from build123d import *

# Parameters (mm, degrees)
F1_DEPTH = 2.4
F2_DEPTH = 8
F3_W     = 64.007707
F3_H     = 6.8
F4_DEPTH = 25
F5_W     = 73.7
F5_H     = 31.871149
F6_DEPTH = 25


with BuildPart() as f1:
    # F0 (on Top) → F1 (new body)
    with BuildSketch(Plane.XY):
        Polygon((-53.5, -17.5), (-53.5, 24.5), (-57.8, 24.5), (-57.8, -17.5), (-57.8, -24.3), (-53.5, -24.3), (53.1, -24.3), (57.8, -24.3), (57.8, -17.5), (53.1, -17.5), align=None)
        Polygon((53.1, 24.5), (-53.5, 24.5), (-53.5, -17.5), (53.1, -17.5), (57.8, -17.5), (57.8, 24.5), align=None)
    extrude(amount=F1_DEPTH)

    # F0 (on Top) → F2 (join)
    with BuildSketch(Plane.XY):
        Polygon((-53.5, -17.5), (-53.5, 24.5), (-57.8, 24.5), (-57.8, -17.5), (-57.8, -24.3), (-53.5, -24.3), (53.1, -24.3), (57.8, -24.3), (57.8, -17.5), (53.1, -17.5), align=None)
    extrude(amount=F2_DEPTH)

    # F3 (on face) → F4 (cut)
    with BuildSketch(Plane.XY.offset(8)):
        with Locations((3.638923, -20.9)):
            Rectangle(F3_W, F3_H)
    extrude(amount=-F4_DEPTH, mode=Mode.SUBTRACT)

    # F5 (on face) → F6 (cut)
    with BuildSketch(Plane.XY.offset(2.4)):
        with Locations((2.150001, 8.564426)):
            Rectangle(F5_W, F5_H)
    extrude(amount=-F6_DEPTH, mode=Mode.SUBTRACT)


solid = f1.part
Could you check a few things on this model? Use its own coordinates, in mm. A direction names the side the tool comes from. Round coordinates to 2 decimals unless told otherwise and drop trailing zeros. Order: outer loops, then holes, each group sorted by start corner. A loop starts at its lowest first (then second) coordinate and runs counter-clockwise, first axis right, second up.
(1) I'm going to push flat-ended pins straight in: pin 1 (1.2 mm diameter, centred on x = 14.5, z = 1, fed in from -Y); pin 2 (8 mm diameter, centred on x = -10.5, y = -18.5, fed in from +Z); pin 3 (1.7 mm diameter, centred on x = -43.5, z = 4, fed in from +Y). Where does each tip first touch, or does it pass through?
Response values:
pin 1: stops at y = -17.5
pin 2: stops at z = 2.4
pin 3: stops at y = -17.5
(2) Imagine slicing it at B-B (z = 5.25). Write out the boundary of the cut face in (x, y).
Response values:
outline: (-57.8, -24.3) - (-28.36, -24.3) - (-28.36, -17.5) - (-53.5, -17.5) - (-53.5, 24.5) - (-57.8, 24.5) - close; (35.64, -24.3) - (57.8, -24.3) - (57.8, -17.5) - (35.64, -17.5) - close
(3) Imagine slicing it at C-C (x = -41). Write out the boundary of the cut face in (y, z).
Response values:
outline: (-24.3, 0) - (24.5, 0) - (24.5, 2.4) - (-17.5, 2.4) - (-17.5, 8) - (-24.3, 8) - close
(4) Which directions (+Z, -Z, +X, -X, +Y, -Y) give clear straight access to the entire face, cutting with the end or side of a thin tool? Please do faces 4 (the flat face through (-49, 24.5, 2)), 5 (the flat face through (35.643, -21, 4)), 6 (the flat face through (39, 8, 1)), 7 (the flat face through (-54, -9, 8)), 8 (the flat face through (-41, -17.5, 5)).
Response values:
face 4: +Z, -Z, +X, -X, +Y
face 5: +Z, -Z, -Y
face 6: +Z, -Z, +Y
face 7: +Z, +X, -X, +Y, -Y
face 8: +Z, +X, +Y
(5) Imagine slicing it at A-A (y = 10.5). Write out the boundary of the cut face in (x, z), plus the area to 3 significant figures.
Response values:
outline: (-57.8, 0) - (-34.7, 0) - (-34.7, 2.4) - (-53.5, 2.4) - (-53.5, 8) - (-57.8, 8) - close; (39, 0) - (57.8, 0) - (57.8, 2.4) - (39, 2.4) - close
area: 125 mm2
(6) Please list where these lines run through material, in increasing order: line 1 along X through (y, z) = (4, 1); line 2 along X through (y, z) = (-20.5, 4.25); line 3 along Y through (x, z) = (-45.5, 5.5).
Response values:
line 1: x = -57.8 to -34.7, 39 to 57.8
line 2: x = -57.8 to -28.36, 35.64 to 57.8
line 3: y = -24.3 to -17.5
(7) Imagine slicing it at D-D (y = -12). Write out the boundary of the cut face in (x, z), plus the area to 3 significant figures.
Response values:
outline: (-57.8, 0) - (57.8, 0) - (57.8, 2.4) - (-53.5, 2.4) - (-53.5, 8) - (-57.8, 8) - close
area: 302 mm2
(8) If we mould it in two halves opening along X, with no side actions, what happens to faces 1 (the flat face through (-11, -10, 2.4)), 2 (the flat face through (-53.5, 3, 5)), 3 (the flat face through (-34.7, 8, 1))? For each: released by +X, released by -X, zero draft, split by the parting line, or undercut.
Response values:
face 1: zero draft
face 2: released by +X
face 3: undercut
